Work out the finished part from the listing and answer in its coordinate system (mm). A direction names the side the tool comes from. Give positions to 0.01 mm unless a question says otherwise; leave off trailing zeros. Loops run counter-clockwise (first coordinate to the right, second up) from the corner with the lowest first, then second, coordinate; pieces in that order, holes last. Notation, with made-up numbers: (29.5, 18.5) -> (36.5, 18.5) arc R17 cw to (36.5, 48.5) -> close; hole circle Ø5 at (-31.5, 25.5). An arc over 180 degrees is marked (long way). Answer as CSV lines item,"result". Start each with the question number.
1. Flat-ended cylindrical pins translate along their axes: pin 1 Ø8 at (x, y) = (-2, 111) entering from -Z; pin 2 Ø8 at (x, z) = (15, 77.5) entering from +Y; pin 3 Ø6 at (x, y) = (10, 149.5) entering from +Z. Find the tip coordinate at first contact, or state that the pin passes through.
2. Determine the mould class of faces 1 (the face through (0.84, 15.07, -11.22)), 2 (the face through (-41, 91, 20)), 3 (the face through (0.84, 25.07, -11.46)), 4 (the face through (1.319, 179.985, 3.238)) for opening direction Y: +Y half, -Y half, draft (parallel to the pull), parting line (faces both ways), or undercut.
3. Find section A-A, the plane x = 0. Give the vertices of the cut face in (y, z), and give its area (3 significant figures).
4. A tool of negligible diameter and unlimited length cuts with its end or side. For faces 5 (the face through (0, 116, 20)), 6 (the face through (-40, 65, 32)), 7 (the face through (1, 40, -17)), 8 (the face through (40, 70, 42)), from which of +Z, -Z, +X, -X, +Y, -Y can it reach the whole face along a straight path? Write none if from no direction.
5. Find the intervals of material crossed by line 1 along Z through (x, y) = (42, 136); line 2 along Z through (x, y) = (-23, 119); line 3 along Y through (x, z) = (3, 24.5), in increasing order.
from build123d import *

# Parameters (mm, degrees)
F0_W      = 120
F0_H      = 40
F1_DEPTH  = 120
F3_DEPTH  = 40
F5_R      = 30
F8_DEPTH  = 77.2940758616
F9_W      = 80
F9_H      = 6
F9_W_2    = 71.5949898127
F10_DEPTH = 120
F6_DEPTH  = 120
F7_DEPTH  = 80


with BuildPart() as f1:
    # F0 (on Front) → F1 (new body)
    with BuildSketch(Plane.XZ):
        Rectangle(F0_W, F0_H)
    extrude(amount=-F1_DEPTH)

    # F2 (on face) → F3 (join)
    with BuildSketch(Plane.XY.offset(20)):
        with BuildLine():
            Line((-60, 120), (60, 120))
            ThreePointArc((60, 120), (0, 180), (-60, 120))
        make_face()
    extrude(amount=-F3_DEPTH)

    # F5 (on face) → F8 (join)
    with BuildSketch(Plane(origin=(0, -8.6602540378, 15), x_dir=(1, 0, 0), z_dir=(0, -0.5, 0.8660254038))):
        with BuildLine():
            Line((-40, 10), (0, 10))
            Line((0, 10), (40, 10))
            Line((40, 10), (40, 110))
            ThreePointArc((40, 110), (0, 70), (-40, 110))
            Line((-40, 110), (-40, 10))
        make_face()
        with BuildLine():
            ThreePointArc((-40, 110), (0, 70), (40, 110))
            ThreePointArc((40, 110), (0, 150), (-40, 110))
        make_face()
        with Locations((0, 110)):
            Circle(F5_R, mode=Mode.SUBTRACT)
    extrude(amount=-F8_DEPTH)

    # F9 (on face) → F10 (cut)
    with BuildSketch(Plane.YZ.offset(60)):
        with Locations((80, -17)):
            Rectangle(F9_W, F9_H)
        with Locations((155.7974949063, -17)):
            Rectangle(F9_W_2, F9_H)
    extrude(amount=-F10_DEPTH, mode=Mode.SUBTRACT)

    # F11 (on face) → F6 (cut)
    with BuildSketch(Plane.YZ.offset(60)):
        Polygon((20, -2.6794919243), (20, -20), (30, -20), align=None)
        Polygon((10, -20), (20, -20), (20, -2.6794919243), align=None)
    extrude(amount=-F6_DEPTH, mode=Mode.SUBTRACT)

    # F7 (cut): a face of the model
    f7_faces = [f1.faces().sort_by_distance(p)[0] for p in [
        (40, 49.0157227063, -28.9795444194),
    ]]
    extrude(f7_faces, amount=-F7_DEPTH, mode=Mode.SUBTRACT)


solid = f1.part
Resolved:
1,pin 1,"stops at z = -14"
1,pin 2,"stops at y = 127.96"
1,pin 3,"stops at z = 43.92"
2,face 1,"undercut"
2,face 2,"draft"
2,face 3,"undercut"
2,face 4,"+Y half"
3,outline,"(0, -20) -> (10, -20) -> (20, -2.68) -> (30, -20) -> (40, -20) -> (40, -14) -> (180, -14) -> (180, 20) -> (154.59, 20) -> (159.89, 23.06) -> (121.24, 90) -> (112.58, 85) -> (150.11, 20) -> (80.83, 20) -> (60.62, 55) -> (0, 20) -> close"
3,area,"8,370 mm^2"
4,face 5,"none"
4,face 6,"+Z, -X, +Y, -Y"
4,face 7,"-Z, +X, -X, +Y"
4,face 8,"+Z, +X, +Y, -Y"
5,line 1,"z = -14 to 20"
5,line 2,"z = -14 to 20, 52.41 to 79.34"
5,line 3,"y = 7.79 to 78.4, 147.34 to 158.93"
